```python
from build123d import *

# Parameters (mm, degrees)
SKETCH2_R   = 9.525
SKETCH2_R_2 = 7.874


with BuildPart() as part:
    # Sweep1: sweep along a path in Sketch1
    with BuildLine(Plane.XY) as sweep1_path:
        Line((28.068079684, 0), (0, 0))
        ThreePointArc((0, 0), (-9.946095847, -0.651901563), (-19.722011237, -2.596452037))
        Line((-19.722011237, -2.596452037), (-73.945377359, -17.1255592))
        ThreePointArc((-73.945377359, -17.1255592), (-83.721292748, -19.070109673), (-93.667388596, -19.722011237))
        Line((-93.667388596, -19.722011237), (-121.735468279, -19.722011237))
    # Sketch2 → Sweep1 (sweep)
    with BuildSketch(Plane.ZY.offset(-28.068079684)):
        Circle(SKETCH2_R)
        Circle(SKETCH2_R_2, mode=Mode.SUBTRACT)
    sweep(path=sweep1_path.line)


solid = part.part
```
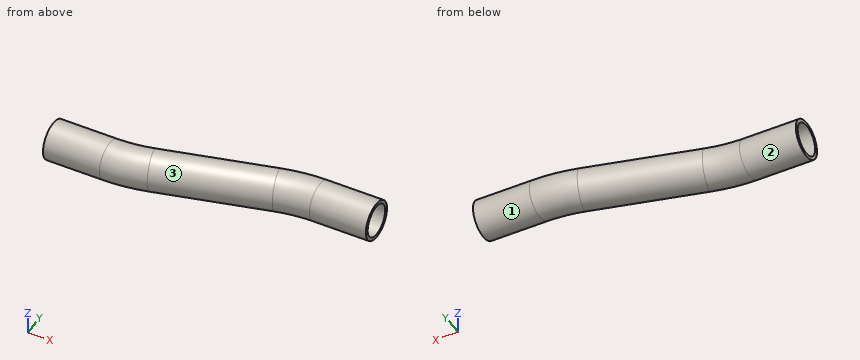
The listing builds one solid part. Answer for the finished solid, in the listing's coordinates (mm). Face numbers are marked on the shaded views. A direction names the side the tool comes from. Coordinates: 2 decimals unless noted, no trailing zeros. Write each loop counter-clockwise with the first axis right and the second up, starting at its lowest first coordinate (ties: lowest second). Pieces come first, ordered by that corner, then holes. Notation, with made-up numbers: (60, 50) - (94, 50) arc R11 ccw to (94, 56) - close; hole circle Ø8 at (9, 11). An arc over 180 degrees is marked (long way). Return JSON: item names as keys, results as strings. Group by question number.
Q1. The part is cut by section A-A on z = 0. Write down the section's boundary in (x, y) (3 decimals), and give its area (3 significant figures).
Q2. Flat-ended cylindrical pins translate along their axes: pin 1 Ø4 at (y, z) = (4, -6.5) entering from +X; pin 2 Ø2 at (x, z) = (-93, 5.5) entering from -Y; pin 3 Ø8 at (x, y) = (-78.5, -24) entering from -Z. Find the tip coordinate at first contact, or state that the pin passes through.
Q3. Find the intervals of material crossed by line 1 along Y through (x, z) = (7.5, 0) (3 decimals); line 2 along Z through (x, y) = (-5, -0.5); line 3 along Y through (x, z) = (-33.5, 6.5), in increasing order. Write a range as [from, to].
Q4. Which of the six approach directions +Z, -Z, +X, -X, +Y, -Y give full straight-line access (tool end or side, diameter ignored) to the marked faces 1, 2 and 3?
Q5. The part is cut by section B-B on x = -109. Write down the section's boundary in (y, z) (3 decimals), and give its area (3 significant figures).
Evaluation:
{
 "1": {"outline": "(-121.735, -29.247) - (-93.667, -29.247) arc R85.725 ccw to (-71.48, -26.326) - (-17.257, -11.797) arc R66.675 cw to (0, -9.525) - (28.068, -9.525) - (28.068, -7.874) - (0, -7.874) arc R68.326 ccw to (-17.684, -10.202) - (-71.907, -24.731) arc R84.074 cw to (-93.667, -27.596) - (-121.735, -27.596) - close; (-121.735, -11.848) - (-93.667, -11.848) arc R68.326 ccw to (-75.983, -9.52) - (-21.76, 5.009) arc R84.074 cw to (0, 7.874) - (28.068, 7.874) - (28.068, 9.525) - (0, 9.525) arc R85.725 ccw to (-22.187, 6.604) - (-76.411, -7.925) arc R66.675 cw to (-93.667, -10.197) - (-121.735, -10.197) - close", "area": "502 mm2"},
 "2": {"pin 1": "stops at x = 28.07", "pin 2": "stops at y = -28.11", "pin 3": "stops at z = -9.37"},
 "3": {"line 1": "y = [-9.525, -7.874], [7.874, 9.525]", "line 2": "z = [-9.52, -7.87], [7.87, 9.52]", "line 3": "y = [-13.5, -10.89], [-1.69, 0.92]"},
 "4": {"face 1": "+X", "face 2": "-X", "face 3": "none"},
 "5": {"outline": "circle Ø19.05 at (-19.722, 0); hole circle Ø15.748 at (-19.722, 0)", "area": "90.2 mm2"}
}
